Verification items for the finished model (mm, model axes). A direction names the side the tool comes from. Round coordinates to 2 decimals unless told otherwise and drop trailing zeros. Write each loop counter-clockwise with the first axis right and the second up, starting at its lowest first coordinate (ties: lowest second). Pieces come first, ordered by that corner, then holes. Notation, with made-up numbers: M 16,67 L 44,67 A34 ccw 44,102 Z; hole C 49,-1 d7. An arc over 180 degrees is marked long. One line per item, written item: value. Start each with the question number.
Item 1: Section check D-D, the plane x = 29.5. Record the cut outline in (y, z).
Item 2: Thickness scan on probe 1 along Y at (x, z) = (8, 37); probe 2 along Y at (x, z) = (33, 30); probe 3 along X at (y, z) = (-15.5, 31). Record the ranges inside material, lowest first. Write a range as from..to.
Item 3: Draft check along X on faces 6 (the face through (5.588, -45, 33)), 7 (the face through (2.755, -31.845, 56.315)), 8 (the face through (45.542, -38, 52)), 9 (the face through (40.462, -38, 52)). Enter one of: +X half, -X half, draft (parallel to the pull), parting line (faces both ways), or undercut.
Item 4: Tool access check on faces 1 (the face through (45.466, -43, 38)), 2 (the face through (25.25, -45.45, 38.14)), 3 (the face through (24, -8, 46.608)), 4 (the face through (24, -8, 29.494)), 5 (the face through (22.41, -23.3, 25.77)). Record the directions out of +Z, -Z, +X, -X, +Y, -Y that give a thin tool (end or side, any length) a straight path to the whole face; none if there is none.
Item 5: Section check A-A, the plane y = -17. Record the cut outline in (x, z), then the cut area to 3 significant figures.
Item 6: Section check C-C, the plane y = -35. Record the cut outline in (x, z), then the cut area to 3 significant figures.
Item 7: Section check B-B, the plane z = 49. Record the cut outline in (x, y), then the cut area to 3 significant figures.
Item 8: Gauge pin test, flat ends, axial feed: pin 1 (11.5 mm diameter, centred on y = -31, z = 43.5, fed in from -X); pin 2 (5 mm diameter, centred on x = 31, y = -33.5, fed in from +Z); pin 3 (17 mm diameter, centred on x = 19, y = -5.5, fed in from -Z); pin 4 (12 mm diameter, centred on x = 32.5, y = -16.5, fed in from +Z). Record the tip position at first contact, or that the pin passes through.
from build123d import *

# Parameters (mm, degrees)
F0_R     = 19.05
F0_R_2   = 16.099385
F1_DEPTH = 5.588
F0_R_3   = 13.139172
F2_DEPTH = 45.466
F4_R     = 19.05
F4_R_2   = 16.099385
F5_DEPTH = 5.08
F6_W     = 20.917241
F6_H     = 17.11411
F7_DEPTH = 15.748


with BuildPart() as f1:
    # F0 (on Right) → F1 (new body)
    with BuildSketch(Plane.YZ):
        with Locations((-29.364781, 37.427243)):
            Circle(F0_R)
        with Locations((-29.364781, 37.427243)):
            Circle(F0_R_2, mode=Mode.SUBTRACT)
    extrude(amount=F1_DEPTH)

    # F0 (on Right) → F2 (join)
    with BuildSketch(Plane.YZ):
        with Locations((-29.364781, 37.427243)):
            Circle(F0_R_2)
        with Locations((-29.364781, 37.427243)):
            Circle(F0_R_3, mode=Mode.SUBTRACT)
    extrude(amount=F2_DEPTH)

    # F4 (on offset) → F5 (join)
    with BuildSketch(Plane.YZ.offset(45.5422)):
        with Locations((-29.376194, 37.433792)):
            Circle(F4_R)
        with Locations((-29.376194, 37.433792)):
            Circle(F4_R_2, mode=Mode.SUBTRACT)
    extrude(amount=-F5_DEPTH)

    # F6 (on Front) → F7 (join)
    with BuildSketch(Plane.XZ):
        with Locations((24.008229, 38.051244)):
            Rectangle(F6_W, F6_H)
    extrude(amount=F7_DEPTH)


solid = f1.part
Response values:
1. outline: M -15.75,46.02 A16.1 ccw long -15.36,29.49 L 0,29.49 L 0,46.61 L -15.75,46.61 Z; hole C -29.36,37.43 d26.28
2. probe 1: y = -45.46..-42.5, -16.23..-13.27
2. probe 2: y = -43.65..-40.2, -18.53..0
2. probe 3: x = 0..45.47
3. face 6: undercut
3. face 7: draft
3. face 8: +X half
3. face 9: undercut
4. face 1: +X
4. face 2: none
4. face 3: +Z, +Y
4. face 4: -Z, +Y
4. face 5: +X, -X
5. outline: M 0,22.94 L 5.59,22.94 L 5.59,27.12 L 40.46,27.12 L 40.46,22.95 L 45.54,22.95 L 45.54,27.14 L 45.47,27.14 L 45.47,32.98 L 0,32.98 Z; M 0,41.87 L 45.47,41.87 L 45.47,47.73 L 45.54,47.73 L 45.54,51.92 L 40.46,51.92 L 40.46,47.74 L 5.59,47.74 L 5.59,51.92 L 0,51.92 Z
5. area: 623 mm2
6. outline: M 0,19.23 L 5.59,19.23 L 5.59,22.35 L 40.46,22.35 L 40.46,19.23 L 45.54,19.23 L 45.54,22.35 L 45.47,22.35 L 45.47,25.56 L 0,25.56 Z; M 0,49.3 L 45.47,49.3 L 45.47,52.51 L 5.59,52.51 L 5.59,55.62 L 0,55.62 Z; M 40.46,52.52 L 45.54,52.52 L 45.54,55.63 L 40.46,55.63 Z
6. area: 359 mm2
7. outline: M 0,-44.5 L 5.59,-44.5 L 5.59,-40.56 L 45.47,-40.56 L 45.47,-35.59 L 0,-35.59 Z; M 0,-23.14 L 45.47,-23.14 L 45.47,-18.18 L 45.54,-18.18 L 45.54,-14.24 L 40.46,-14.24 L 40.46,-18.17 L 5.59,-18.17 L 5.59,-14.23 L 0,-14.23 Z; M 40.46,-44.51 L 45.54,-44.51 L 45.54,-40.57 L 40.46,-40.57 Z
7. area: 536 mm2
8. pin 1: passes through
8. pin 2: stops at z = 53.44
8. pin 3: stops at z = 29.49
8. pin 4: stops at z = 51.99
